Model file for the job. Use its own axes, mm. Face numbers are marked on the shaded views. Coordinates: 2 decimals unless noted, no trailing zeros. Loops run counter-clockwise (first coordinate to the right, second up) from the corner with the lowest first, then second, coordinate; pieces in that order, holes last. Notation, with made-up numbers: (78, -22.5) -> (84, -22.5) arc R24 cw to (84, 11.5) -> close; hole circle Ø3 at (-1, -0.75). An arc over 180 degrees is marked (long way). Use one line per item in the form item = value.
```python
from build123d import *

# Parameters (mm, degrees)
F0_R      = 7
F1_DEPTH  = 7
F2_R      = 6.99999
F4_DEPTH  = 40
F5_R      = 7
F5_R_2    = 5.75
F6_DEPTH  = 1.5
F7_R      = 7
F7_R_2    = 5.1
F8_DEPTH  = 12.9
F10_DEPTH = 1


# Not quite as in the source:
# - a fillet or chamfer is up to 0.001 mm smaller than in the source, because OpenCascade refuses the exact size


with BuildPart() as f1:
    # F0 (on Top) → F1 (new body)
    with BuildSketch(Plane.XY):
        Circle(F0_R)
        with BuildLine():
            ThreePointArc((-5.75, 0), (0, 5.75), (5.75, 0))
            ThreePointArc((5.75, 0), (0, -5.75), (-5.75, 0))
        make_face(mode=Mode.SUBTRACT)
        with BuildLine():
            Line((-5.75, 0), (5.75, 0))
            ThreePointArc((5.75, 0), (0, 5.75), (-5.75, 0))
        make_face()
        with BuildLine():
            ThreePointArc((-5.75, 0), (0, -5.75), (5.75, 0))
            Line((5.75, 0), (-5.75, 0))
        make_face()
    extrude(amount=-F1_DEPTH)

    # F2 (radius 7 in the source; OpenCascade refuses exactly that, so slightly less here)
    f2_edges = [f1.edges().sort_by_distance(p)[0] for p in [
        (-7, 0, -7),
    ]]
    fillet(f2_edges, radius=F2_R)

    # F0 (on Top) → F3 (revolve, cut)
    with BuildSketch(Plane.XY):
        with BuildLine():
            ThreePointArc((-5.75, 0), (0, -5.75), (5.75, 0))
            Line((5.75, 0), (-5.75, 0))
        make_face()
    revolve(axis=Axis((0, 0, 0), (1, 0, 0)), mode=Mode.SUBTRACT)

    # F4 (add): a face of the model
    f4_faces = [f1.faces().sort_by_distance(p)[0] for p in [
        (-6.8020101013, 0, 0),
    ]]
    extrude(f4_faces, amount=F4_DEPTH)

    # F5 (on face) → F6 (join)
    with BuildSketch(Plane.XY.offset(40)):
        Circle(F5_R)
        Circle(F5_R_2, mode=Mode.SUBTRACT)
        Circle(F5_R_2)
    extrude(amount=F6_DEPTH)

    # F7 (on face) → F8 (join)
    with BuildSketch(Plane.XY.offset(41.5)):
        Circle(F7_R)
        Circle(F7_R_2, mode=Mode.SUBTRACT)
    extrude(amount=F8_DEPTH)

    # F9 (on face) → F10 (join)
    with BuildSketch(Plane.XY.offset(54.4)):
        with BuildLine():
            ThreePointArc((-6.6038061512, -2.3215822875), (-6.9002406863, -1.1775731276), (-7, 0))
            Line((-7, 0), (-10.0409816951, 0))
            Line((-10.0409816951, 0), (-10.0409816951, 7.0408415049))
            Line((-10.0409816951, 7.0408415049), (-27.5440905243, 7.0408415049))
            Line((-27.5440905243, 7.0408415049), (-27.5440905243, -6.5598203801))
            Line((-27.5440905243, -6.5598203801), (-27.5440905243, -8.1330426037))
            Line((-27.5440905243, -8.1330426037), (-9.7872372717, -8.1330426037))
            Line((-9.7872372717, -8.1330426037), (-9.7872372717, -2.3215822875))
            Line((-9.7872372717, -2.3215822875), (-6.6038061512, -2.3215822875))
        make_face()
        with BuildLine():
            Line((-0.5746171277, 9.2485286327), (-0.5746171277, 6.9763755028))
            ThreePointArc((-0.5746171277, 6.9763755028), (0.5741414209, 6.9764146686), (1.7074374482, 6.7885681377))
            Line((1.7074374482, 6.7885681377), (1.7074374482, 9.2485286327))
            Line((1.7074374482, 9.2485286327), (11.8826339021, 9.2485286327))
            Line((11.8826339021, 9.2485286327), (11.8826339021, 21.6566864401))
            Line((11.8826339021, 21.6566864401), (-10.5484733358, 21.6566864401))
            Line((-10.5484733358, 21.6566864401), (-10.5484733358, 9.2485286327))
            Line((-10.5484733358, 9.2485286327), (-7.0214094594, 9.2485286327))
            Line((-7.0214094594, 9.2485286327), (-0.5746171277, 9.2485286327))
        make_face()
        with BuildLine():
            Line((14.655204518, 0.8017900982), (6.9539292949, 0.8017900982))
            ThreePointArc((6.9539292949, 0.8017900982), (6.9884728326, 0.4015563072), (7, 0))
            ThreePointArc((7, 0), (6.9335784443, -0.9620238859), (6.735574298, -1.9057908794))
            Line((6.735574298, -1.9057908794), (19.9458785355, -1.9057908794))
            Line((19.9458785355, -1.9057908794), (19.9458785355, -11.5896631032))
            Line((19.9458785355, -11.5896631032), (38.256034255, -11.5896631032))
            Line((38.256034255, -11.5896631032), (38.256034255, 13.5597093031))
            Line((38.256034255, 13.5597093031), (19.1134941834, 13.5597093031))
            Line((19.1134941834, 13.5597093031), (19.1134941834, 0.8017900982))
            Line((19.1134941834, 0.8017900982), (14.655204518, 0.8017900982))
        make_face()
        with BuildLine():
            ThreePointArc((1.6340564471, -6.8066041113), (0.3847522235, -6.989418125), (-0.8770696547, -6.9448361263))
            Line((-0.8770696547, -6.9448361263), (-0.8770696547, -9.9506975346))
            Line((-0.8770696547, -9.9506975346), (-10.5280578136, -9.9506975346))
            Line((-10.5280578136, -9.9506975346), (-10.5280578136, -24.5994888246))
            Line((-10.5280578136, -24.5994888246), (15.0621160865, -24.5994888246))
            Line((15.0621160865, -24.5994888246), (15.0621160865, -10.4480329901))
            Line((15.0621160865, -10.4480329901), (1.6340564471, -10.4480329901))
            Line((1.6340564471, -10.4480329901), (1.6340564471, -6.8066041113))
        make_face()
    extrude(amount=-F10_DEPTH)


solid = f1.part
```
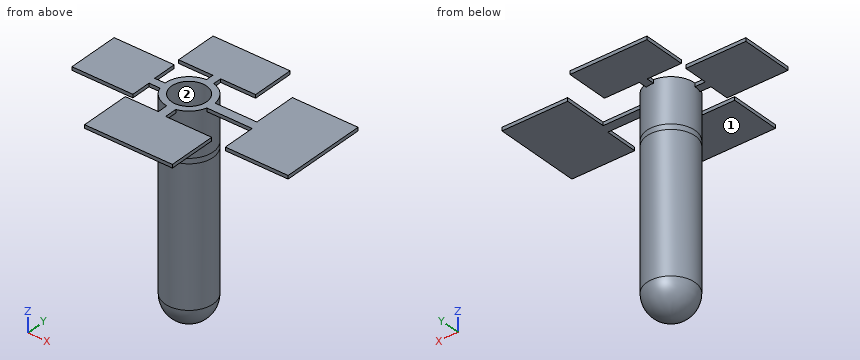
Q1. Pin check, flat tips, straight feed: pin 1 Ø10 at (y, z) = (3, 0.5) entering from +X; pin 2 Ø12 at (x, y) = (4, 11.5) entering from -Z; pin 3 Ø1.1 at (y, z) = (9, 53.5) entering from -X; pin 4 Ø9 at (x, y) = (-2, -2) entering from -Z. Stop position of each tip, or through.
Result:
pin_1 = 7
pin_2 = -3.3
pin_3 = -10.55
pin_4 = -7
Q2. Band-saw the part on A-A, the plane z = 5. Write the cut outline in (x, y).
Result:
outline = circle Ø14 at (0, 0); hole circle Ø11.5 at (0, 0)
Q3. Band-saw the part on B-B, the plane y = 17. Write the cut outline in (x, z).
Result:
outline = (-10.55, 53.4) -> (11.88, 53.4) -> (11.88, 54.4) -> (-10.55, 54.4) -> close
Q4. Mould opens along Y. For the marked faces 1 and 2 say: released by +Y, released by -Y, zero draft, split by the parting line, or undercut.
Result:
face_1 = zero draft
face_2 = undercut
Q5. Band-saw the part on C-C, the plane x = 18. Write the cut outline in (y, z), and give its area (3 significant figures).
Result:
outline = (-1.91, 53.4) -> (0.8, 53.4) -> (0.8, 54.4) -> (-1.91, 54.4) -> close
area = 2.71 mm2
Q6. Wall check: line 1 along Y through (x, z) = (0, 31); line 2 along Z through (x, y) = (34.5, 1.5); line 3 along Y through (x, z) = (0, 50). Give the ranges that are in metal, low to high.
Result:
line_1 = -7 to -5.75, 5.75 to 7
line_2 = 53.4 to 54.4
line_3 = -7 to -5.1, 5.1 to 7
